The figure shows three views and two pictorial views of one solid part (mm, origin at its lowest corner). Answer the questions. A direction names the side the tool comes from. Round coordinates to 2 decimals unless told otherwise and drop trailing zeros. Write each loop counter-clockwise with the first axis right and the second up, starting at its lowest first coordinate (ties: lowest second). Pieces come first, ordered by that corner, then holes. Notation, with made-up numbers: M 76.5,33.5 L 101.5,33.5 A34 ccw 101.5,64.5 Z; hole C 39,-3.5 d3. An arc over 180 degrees is marked long. One line per item, written item: value. Start each with the question number.
Q1. Find section C-C (x = 40.5). Write down the section's boundary in (y, z), and give its area (3 significant figures).
Q2. A tool of negligible diameter and unlimited length cuts with its end or side. For the marked faces 1, 2, 3, 4 and 5, from which of +Z, -Z, +X, -X, +Y, -Y can it reach the whole face along a straight path? Write none if from no direction.
Q3. Find section D-D (y = 12.5). Write down the section's boundary in (x, z).
Q4. Find section B-B (z = 24). Write down the section's boundary in (x, y), and give its area (3 significant figures).
Q5. The mould has two halves that part along Z. Classify the marked faces 6, 7, 8 and 9: released by +Z, released by -Z, zero draft, split by the parting line, or undercut.
Q6. Given pin 1 Ø7.5 at (y, z) = (8, 24.5) entering from +X; pin 2 Ø12.5 at (x, y) = (25.5, 15.5) entering from +Z; pin 3 Ø4 at (x, y) = (20.5, 8.5) entering from -Z, each flat-ended and moving along its own axis, determine where each tip first touches the part or whether it passes through.
Q7. Consider probe 1 along Z at (x, y) = (34.5, 49.5); probe 2 along Y at (x, z) = (7, 38); probe 3 along Y at (x, z) = (26.5, 23). Determine where each line is inside the solid, lowest interval first.
Q8. Find section A-A (y = 43.5). Write down the section's boundary in (x, z).
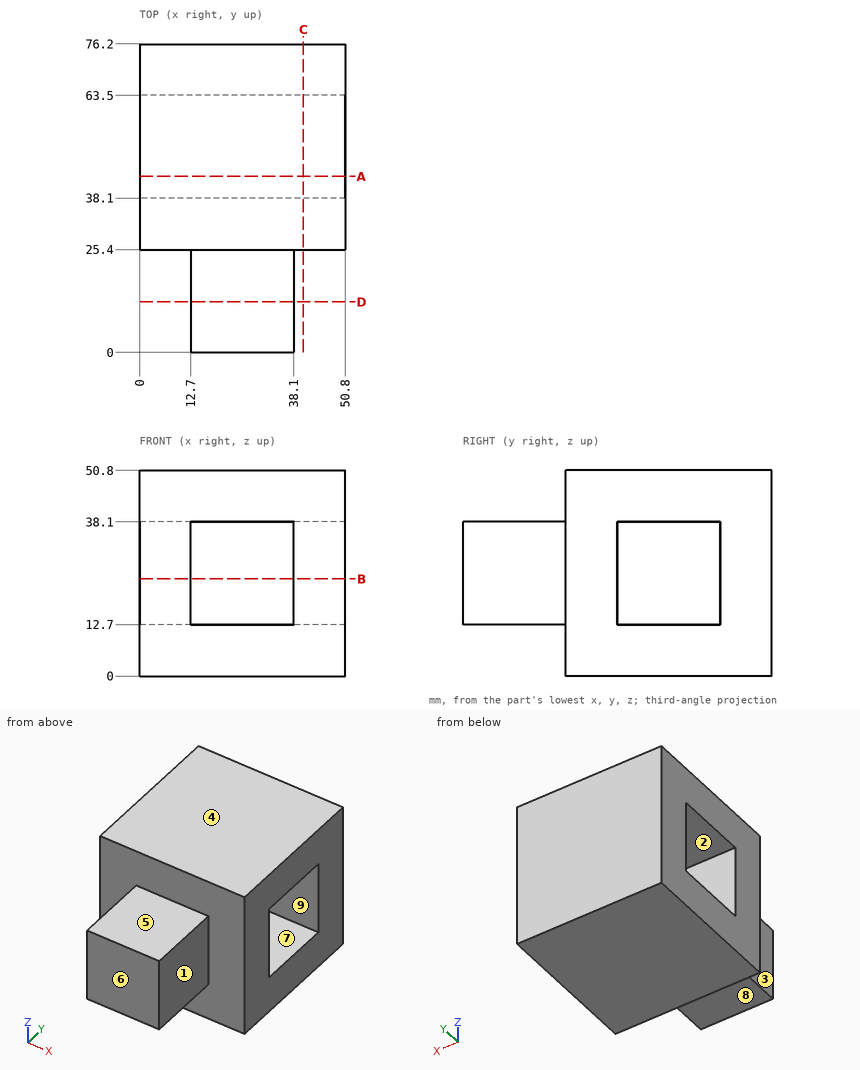
The answers:
1. outline: M 25.4,0 L 76.2,0 L 76.2,50.8 L 25.4,50.8 Z; hole M 38.1,12.7 L 63.5,12.7 L 63.5,38.1 L 38.1,38.1 Z
1. area: 1,940 mm2
2. face 1: +Z, -Z, +X, -Y
2. face 2: +X, -X
2. face 3: +Z, -Z, -X, -Y
2. face 4: +Z, +X, -X, +Y, -Y
2. face 5: +Z, +X, -X, -Y
3. outline: M 12.7,12.7 L 38.1,12.7 L 38.1,38.1 L 12.7,38.1 Z
4. outline: M 0,25.4 L 12.7,25.4 L 12.7,0 L 38.1,0 L 38.1,25.4 L 50.8,25.4 L 50.8,38.1 L 0,38.1 Z; M 0,63.5 L 50.8,63.5 L 50.8,76.2 L 0,76.2 Z
4. area: 1,940 mm2
5. face 6: zero draft
5. face 7: undercut
5. face 8: released by -Z
5. face 9: undercut
6. pin 1: x = 38.1
6. pin 2: z = 38.1
6. pin 3: z = 12.7
7. probe 1: 0 to 12.7, 38.1 to 50.8
7. probe 2: 25.4 to 38.1, 63.5 to 76.2
7. probe 3: 0 to 38.1, 63.5 to 76.2
8. outline: M 0,0 L 50.8,0 L 50.8,12.7 L 0,12.7 Z; M 0,38.1 L 50.8,38.1 L 50.8,50.8 L 0,50.8 Z
